Could you check a few things on this model? Use its own coordinates, in mm. Face numbers are marked on the shaded views. A direction names the side the tool comes from. Give positions to 0.01 mm unless a question says otherwise; leave off trailing zeros. Order: outer loops, then holes, each group sorted by start corner. A loop starts at its lowest first (then second) coordinate and runs counter-clockwise, first axis right, second up. Notation, with made-up numbers: M 22.5,45 L 60.5,45 A16 cw 60.5,56 Z; hole C 76,78.5 d8. An arc over 180 degrees is marked long. Use a Markdown table: item, result. Add a question column.
Item 1: Suppose I cut it at B-B on y = 40. Write out the boundary of the cut face in (x, z), plus the area to 3 significant figures.
Item 2: For the marked faces 5 and 6, which set-ups out of +Z, -Z, +X, -X, +Y, -Y let a thin tool reach every point of the face, with its end or its side?
Item 3: Suppose I cut it at D-D on z = -2.75. Write out the boundary of the cut face in (x, y).
Item 4: If we mould it in two halves opening along Z, with no side actions, what happens to the marked faces 1, 2, 3 and 4? For each: released by +Z, released by -Z, zero draft, split by the parting line, or undercut.
Item 5: Suppose I cut it at A-A on x = 0. Write out the boundary of the cut face in (y, z), plus the area to 3 significant figures.
Item 6: If I drill on L1, parallel to X at y = 36, z = 0; L2, parallel to Z at x = 0, y = 37; L3, parallel to Y at x = 0.25, z = -1, over which ranges is the centre line in solid material (lowest first)? Write a range as from..to.
Item 7: I'm going to push flat-ended pins straight in: pin 1 Ø3 at (x, z) = (-1, 2.5) entering from -Y; pin 2 Ø2.5 at (x, z) = (-1.5, 0) entering from +Y; pin 3 Ø4 at (y, z) = (9, 2.5) entering from +X; pin 4 Ø3 at (x, z) = (0, 0) entering from +Y. Where does each tip first touch, or does it pass through?
Item 8: Suppose I cut it at C-C on y = 32. Write out the boundary of the cut face in (x, z).
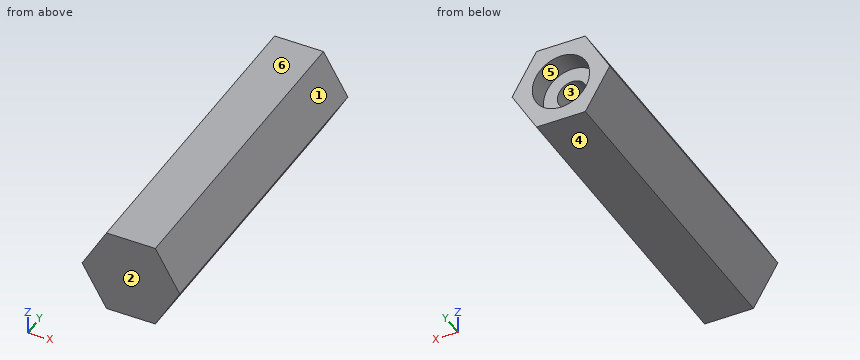
from build123d import *

# Parameters (mm, degrees)
SALIENTE_EXTRUIR1_DEPTH = 45
CROQUIS2_R              = 4
CORTAR_EXTRUIR1_DEPTH   = 3
CROQUIS3_R              = 2.05
CORTAR_EXTRUIR2_DEPTH   = 11
SALIENTE_EXTRUIR2_DEPTH = 11


with BuildPart() as part:
    # Croquis1 → Saliente-Extruir1 (new body)
    with BuildSketch(Plane(origin=(0, 0, 0), x_dir=(1, 0, 0), z_dir=(0, 1, 0))):
        Polygon((6.812733176, 0), (3.406366588, 5.9), (-3.406366588, 5.9), (-6.812733176, 0), (-3.406366588, -5.9), (3.406366588, -5.9), align=None)
    extrude(amount=SALIENTE_EXTRUIR1_DEPTH)

    # Croquis2 → Cortar-Extruir1 (cut)
    with BuildSketch(Plane(origin=(0, 45, 0), x_dir=(1, 0, 0), z_dir=(0, 1, 0))):
        with Locations(Location((0, 0, 0), (0, 0, 270))):
            Circle(CROQUIS2_R)
    extrude(amount=-CORTAR_EXTRUIR1_DEPTH, mode=Mode.SUBTRACT)

    # Croquis3 → Cortar-Extruir2 (cut)
    with BuildSketch(Plane(origin=(0, 42, 0), x_dir=(1, 0, 0), z_dir=(0, 1, 0))):
        with Locations(Location((0, 0, 0), (0, 0, 270))):
            Circle(CROQUIS3_R)
    extrude(amount=-CORTAR_EXTRUIR2_DEPTH, mode=Mode.SUBTRACT)

    # Croquis4 → Saliente-Extruir2 (add)
    with BuildSketch(Plane(origin=(0, 39.5, 0), x_dir=(1, 0, 0), z_dir=(0, 1, 0))):
        with BuildLine():
            Line((-1.449137675, 1.45), (1.449137675, 1.45))
            ThreePointArc((1.449137675, 1.45), (0, 2.05), (-1.449137675, 1.45))
        make_face()
    extrude(amount=-SALIENTE_EXTRUIR2_DEPTH)


solid = part.part
Findings below:
| question | item | result |
|---|---|---|
| 1 | outline | M -6.81,0 L -3.41,-5.9 L 3.41,-5.9 L 6.81,0 L 3.41,5.9 L -3.41,5.9 Z; hole C 0,0 d4.1 |
| 1 | area | 107 mm^2 |
| 2 | face 5 | +Y |
| 2 | face 6 | +Z, +X, -X, +Y, -Y |
| 3 | outline | M -5.23,0 L 5.23,0 L 5.23,45 L 2.9,45 L 2.9,42 L -2.9,42 L -2.9,45 L -5.23,45 Z |
| 4 | face 1 | released by +Z |
| 4 | face 2 | zero draft |
| 4 | face 3 | undercut |
| 4 | face 4 | released by -Z |
| 5 | outline | M 0,-5.9 L 45,-5.9 L 45,-4 L 42,-4 L 42,-2.05 L 39.5,-2.05 L 39.5,-1.45 L 31,-1.45 L 31,2.05 L 42,2.05 L 42,4 L 45,4 L 45,5.9 L 0,5.9 Z |
| 5 | area | 467 mm^2 |
| 6 | L1 | x = -6.81..-2.05, 2.05..6.81 |
| 6 | L2 | z = -5.9..-1.45, 2.05..5.9 |
| 6 | L3 | y = 0..31 |
| 7 | pin 1 | stops at y = 0 |
| 7 | pin 2 | stops at y = 42 |
| 7 | pin 3 | stops at x = 6.52 |
| 7 | pin 4 | stops at y = 39.5 |
| 8 | outline | M -6.81,0 L -3.41,-5.9 L 3.41,-5.9 L 6.81,0 L 3.41,5.9 L -3.41,5.9 Z; hole M -1.45,-1.45 L 1.45,-1.45 A2.05 ccw long Z |
